Design review of the part built by this model. Coordinates are the model's own, in mm. Give positions to 0.01 mm unless a question says otherwise; leave off trailing zeros. Write each loop counter-clockwise with the first axis right and the second up, starting at its lowest first coordinate (ties: lowest second). Pieces come first, ordered by that corner, then holes. Notation, with made-up numbers: M 87,-18 L 131,-18 A20 ccw 131,7 Z; hole C 52.5,67 d6. An arc over 180 degrees is marked long. Answer in a Markdown table with one row per item.
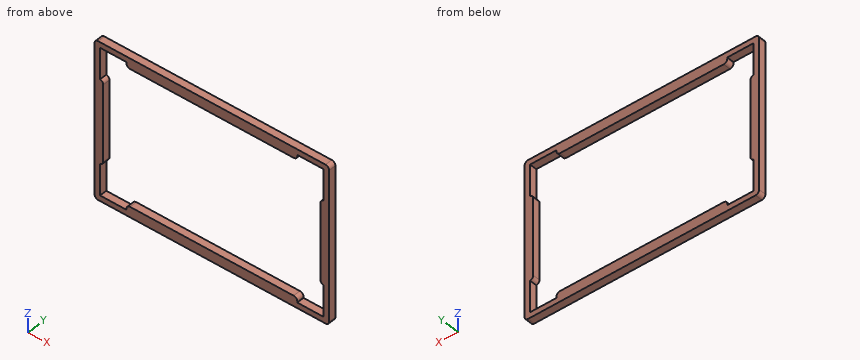
```python
from build123d import *

# Parameters (mm, degrees)
SKETCH2_W           = 127.76
SKETCH2_H           = 85.48
SKETCH2_W_2         = 121.76
SKETCH2_H_2         = 79.48
SKETCH2_W_3         = 1.73
SKETCH2_H_3         = 45.5
SKETCH2_W_4         = 93
SKETCH2_H_4         = 2.65
BOSS_EXTRUDE1_DEPTH = 4
FILLET1_R           = 2


with BuildPart() as part:
    # Sketch2 → Boss-Extrude1 (new body)
    # profile 1 of 5: a face of its own
    with BuildSketch(Plane(origin=(0, 0, 0), x_dir=(1, 0, 0), z_dir=(0, 1, 0))):
        Rectangle(SKETCH2_W, SKETCH2_H)
        Rectangle(SKETCH2_W_2, SKETCH2_H_2, mode=Mode.SUBTRACT)
    # profile 2 of 5: a face of its own
    with BuildSketch(Plane(origin=(0, 0, 0), x_dir=(1, 0, 0), z_dir=(0, 1, 0))):
        with Locations((-60.015, 0)):
            Rectangle(SKETCH2_W_3, SKETCH2_H_3)
    # profile 3 of 5: a face of its own
    with BuildSketch(Plane(origin=(0, 0, 0), x_dir=(1, 0, 0), z_dir=(0, 1, 0))):
        with Locations((0, 38.415)):
            Rectangle(SKETCH2_W_4, SKETCH2_H_4)
    # profile 4 of 5: a face of its own
    with BuildSketch(Plane(origin=(0, 0, 0), x_dir=(1, 0, 0), z_dir=(0, 1, 0))):
        with Locations((60.015, 0)):
            Rectangle(SKETCH2_W_3, SKETCH2_H_3)
    # profile 5 of 5: a face of its own
    with BuildSketch(Plane(origin=(0, 0, 0), x_dir=(1, 0, 0), z_dir=(0, 1, 0))):
        with Locations((0, -38.415)):
            Rectangle(SKETCH2_W_4, SKETCH2_H_4)
    extrude(amount=BOSS_EXTRUDE1_DEPTH)

    # Fillet1
    # the kernel refuses this fillet: 2 mm, written as the material it takes off along each edge
    with BuildSketch(Plane(origin=(46.5, -5, 37.09), x_dir=(0, 0, 1), z_dir=(0, 1, 0)), Plane(origin=(-46.5, -5, 37.09), x_dir=(1, 0, 0), z_dir=(0, 1, 0)), Plane(origin=(-63.88, -5, 42.74), x_dir=(0, 0, -1), z_dir=(0, 1, 0)), Plane(origin=(63.88, -5, 42.74), x_dir=(-1, 0, 0), z_dir=(0, 1, 0))) as fillet1_piece_1:
        with BuildLine():
            CenterArc((FILLET1_R, -FILLET1_R), FILLET1_R, 90, 90)
            Line((0, -FILLET1_R), (-FILLET1_R * 0.02, -FILLET1_R))
            Line((-FILLET1_R * 0.02, -FILLET1_R), (-FILLET1_R * 0.02, FILLET1_R * 0.02))
            Line((-FILLET1_R * 0.02, FILLET1_R * 0.02), (FILLET1_R, FILLET1_R * 0.02))
            Line((FILLET1_R, FILLET1_R * 0.02), (FILLET1_R, 0))
        make_face()
    extrude(amount=14, mode=Mode.SUBTRACT)
    with BuildSketch(Plane(origin=(59.15, -4.954227992, 22.75), x_dir=(1, 0, 0), z_dir=(0, 1, 0)), Plane(origin=(-59.15, -4.954227992, -22.75), x_dir=(-1, 0, 0), z_dir=(0, 1, 0))) as fillet1_piece_2:
        with BuildLine():
            CenterArc((2, 1.981691197), FILLET1_R, 180, 82.241380111)
            Line((0, 1.981691197), (-0.04, 1.981691197))
            Line((-0.04, 1.981691197), (-0.04, 0))
            Line((-0.04, 0), (0, -0.04))
            ThreePointArc((0, -0.04), (0.865, -0.04), (1.7246, -0.039633824))
            Line((1.7246, -0.039633824), (1.73, 0))
        make_face()
    extrude(amount=13.908455985, mode=Mode.SUBTRACT)
    with BuildSketch(Plane(origin=(59.15, -4.954227992, -22.75), x_dir=(0, 0, 1), z_dir=(0, 1, 0)), Plane(origin=(-59.15, -4.954227992, 22.75), x_dir=(0, 0, -1), z_dir=(0, 1, 0))) as fillet1_piece_3:
        with BuildLine():
            CenterArc((1.981691197, 2), FILLET1_R, 187.758619889, 82.241380111)
            Line((0, 1.73), (-0.039633824, 1.7246))
            ThreePointArc((-0.039633824, 1.7246), (-0.04, 0.865), (-0.04, 0))
            Line((-0.04, 0), (0, -0.04))
            Line((0, -0.04), (1.981691197, -0.04))
            Line((1.981691197, -0.04), (1.981691197, 0))
        make_face()
    extrude(amount=13.908455985, mode=Mode.SUBTRACT)
    with BuildSketch(Plane(origin=(46.5, -5, -37.09), x_dir=(0, 0, -1), z_dir=(0, 1, 0)), Plane(origin=(-46.5, -5, -37.09), x_dir=(1, 0, 0), z_dir=(0, 1, 0)), Plane(origin=(-63.88, -5, -42.74), x_dir=(0, 0, 1), z_dir=(0, 1, 0)), Plane(origin=(63.88, -5, -42.74), x_dir=(-1, 0, 0), z_dir=(0, 1, 0))) as fillet1_piece_4:
        with BuildLine():
            CenterArc((FILLET1_R, FILLET1_R), FILLET1_R, 180, 90)
            Line((0, FILLET1_R), (-FILLET1_R * 0.02, FILLET1_R))
            Line((-FILLET1_R * 0.02, FILLET1_R), (-FILLET1_R * 0.02, -FILLET1_R * 0.02))
            Line((-FILLET1_R * 0.02, -FILLET1_R * 0.02), (FILLET1_R, -FILLET1_R * 0.02))
            Line((FILLET1_R, -FILLET1_R * 0.02), (FILLET1_R, 0))
        make_face()
    extrude(amount=14, mode=Mode.SUBTRACT)


solid = part.part
```
1) To check wall thickness, follow probe 1 along X at (y, z) = (1.15, -27); probe 2 along X at (y, z) = (0.3, -13.5); probe 3 along Z at (x, y) = (-17, 0.4). State the ranges of each line that lie inside material, in increasing order. Write a range as [from, to].
Geometry says:
| item | result |
|---|---|
| probe 1 | [-63.88, -60.88], [60.88, 63.88] |
| probe 2 | [-63.88, -59.15], [59.15, 63.88] |
| probe 3 | [-42.74, -37.09], [37.09, 42.74] |
2) Add section B-B (x = -49.5). Write out the cut boundary in (y, z).
Geometry says:
| item | result |
|---|---|
| outline | M 0,-42.74 L 4,-42.74 L 4,-39.74 L 0,-39.74 Z; M 0,39.74 L 4,39.74 L 4,42.74 L 0,42.74 Z |
3) Add section A-A (z = -24.5). Write out the cut boundary in (x, y), and give its area (3 significant figures).
Geometry says:
| item | result |
|---|---|
| outline | M -63.88,0 L -60.88,0 L -60.88,4 L -63.88,4 Z; M 60.88,0 L 63.88,0 L 63.88,4 L 60.88,4 Z |
| area | 24.0 mm^2 |
